```python
from build123d import *

# Parameters (mm, degrees)
SKETCH_1_R      = 1.5
EXTRUDE_1_DEPTH = 3
FILLET_4_R      = 5


with BuildPart() as part:
    # 草图1 → 凸台-拉伸1 (new body)
    with BuildSketch(Plane(origin=(0, 0, 0), x_dir=(1, 0, 0), z_dir=(0, 1, 0))):
        with BuildLine():
            Line((-33, 0), (-33, 67))
            Line((-33, 67), (-39.23, 78.185494034))
            Line((-39.23, 78.185494034), (-45.46, 67))
            Line((-45.46, 67), (-45.46, -42.262061372))
            Line((-45.46, -42.262061372), (-10.274300832, -42.262061372))
            Line((-10.274300832, -42.262061372), (-10.274300832, -31.359826887))
            ThreePointArc((-10.274300832, -31.359826887), (-26.721264261, -19.364246339), (-33, 0))
        make_face()
        with Locations(Location((-31.96, -34.222061372, 0), (0, 0, 270))):
            Circle(SKETCH_1_R, mode=Mode.SUBTRACT)
    extrude(amount=EXTRUDE_1_DEPTH)

    # 圆角4
    fillet_4_edges = [part.edges().sort_by_distance(p)[0] for p in [
        (-39.23, 1.5, -78.185494034),
    ]]
    fillet(fillet_4_edges, radius=FILLET_4_R)


solid = part.part
```
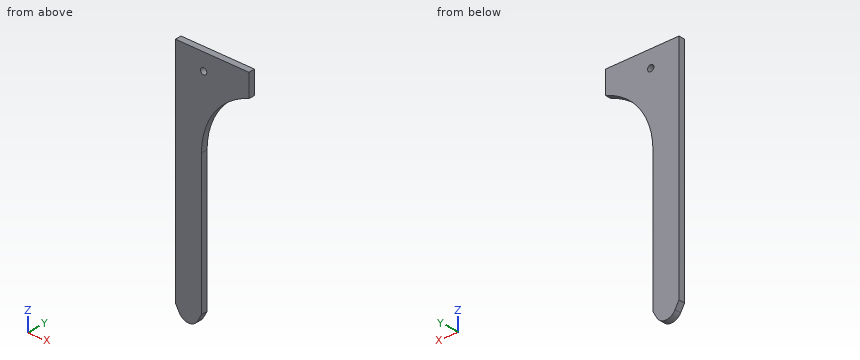
Build history of the part. All positions in model axes, mm. Round coordinates to 2 decimals unless told otherwise and drop trailing zeros. Order: outer loops, then holes, each group sorted by start corner. A loop starts at its lowest first (then second) coordinate and runs counter-clockwise, first axis right, second up. Notation, with made-up numbers: (55.25, -23) -> (60.25, -23) arc R19 cw to (60.25, 12) -> close; hole circle Ø8 at (24, 64.25). An arc over 180 degrees is marked (long way). Answer in a Markdown table with one row per item.
1) Pin check, flat tips, straight feed: P1, Ø12, axis at x = -22.5, z = 13.5, coming from the +Y side; P2, Ø1, axis at y = 2, z = 0.5, coming from the +X side. Stop position of each tip, or through.
Values:
| item | result |
|---|---|
| P1 | through |
| P2 | x = -32.98 |
2) Band-saw the part on C-C on z = -39. Give the cut face in (x, y), and give its area (3 significant figures).
Values:
| item | result |
|---|---|
| outline | (-45.46, 0) -> (-33, 0) -> (-33, 3) -> (-45.46, 3) -> close |
| area | 37.4 mm2 |
3) Band-saw the part on B-B on x = -31.96. Give the cut face in (y, z), and give its area (3 significant figures).
Values:
| item | result |
|---|---|
| outline | (0, 8.22) -> (3, 8.22) -> (3, 32.72) -> (0, 32.72) -> close; (0, 35.72) -> (3, 35.72) -> (3, 42.26) -> (0, 42.26) -> close |
| area | 93.1 mm2 |
4) Band-saw the part on A-A on y = 1.4. Give the cut face in (x, z).
Values:
| item | result |
|---|---|
| outline | (-45.46, -67) -> (-43.6, -70.34) arc R5 ccw to (-34.86, -70.34) -> (-33, -67) -> (-33, 0) arc R33 cw to (-10.27, 31.36) -> (-10.27, 42.26) -> (-45.46, 42.26) -> close; hole circle Ø3 at (-31.96, 34.22) |
5) Wall check: L1, parallel to X at y = 0.9, z = -58.5; L2, parallel to X at y = 1.55, z = 7; L3, parallel to Z at x = -28, y = 2.7. Give the ranges that are in metal, low to high.
Values:
| item | result |
|---|---|
| L1 | -45.46 to -33 |
| L2 | -45.46 to -32.25 |
| L3 | 17.46 to 42.26 |
6) Band-saw the part on D-D on x = -22.5. Give the cut face in (y, z), and give its area (3 significant figures).
Values:
| item | result |
|---|---|
| outline | (0, 24.14) -> (3, 24.14) -> (3, 42.26) -> (0, 42.26) -> close |
| area | 54.4 mm2 |
